Can you work these out from the model? Positions are in its coordinate system, mm. Coordinates: 2 decimals unless noted, no trailing zeros. Write each loop counter-clockwise with the first axis right and the second up, starting at its lowest first coordinate (ties: lowest second). Pieces come first, ordered by that corner, then holes.
```python
from build123d import *

# Parameters (mm, degrees)
SKETCH2_R           = 6.35
SKETCH2_R_2         = 3.175
SKETCH2_R_3         = 10.9855
BOSS_EXTRUDE1_DEPTH = 4.445
SKETCH4_R           = 3.175
CUT_EXTRUDE2_DEPTH  = 148.450257689
SKETCH6_W           = 63.5
SKETCH6_H           = 2.797978373
CUT_EXTRUDE3_DEPTH  = 148.450257689


with BuildPart() as part:
    # Sketch2 → Boss-Extrude1 (new body)
    with BuildSketch(Plane.XY):
        with BuildLine():
            Line((31.75, 112.17275), (-31.75, 112.17275))
            Line((-31.75, 112.17275), (-31.75, 52.48275))
            ThreePointArc((-31.75, 52.48275), (-12.7, -17.145), (-31.75, -86.77275))
            Line((-31.75, -86.77275), (-31.75, -112.17275))
            ThreePointArc((-31.75, -112.17275), (0, -143.92275), (31.75, -112.17275))
            Line((31.75, -112.17275), (31.75, -86.77275))
            ThreePointArc((31.75, -86.77275), (12.7, -17.145), (31.75, 52.48275))
            Line((31.75, 52.48275), (31.75, 112.17275))
        make_face()
        with Locations((0, -112.17275)):
            Circle(SKETCH2_R, mode=Mode.SUBTRACT)
        with Locations((-22.86, 79.15275)):
            Circle(SKETCH2_R_2, mode=Mode.SUBTRACT)
        with Locations((0, 65.18275)):
            Circle(SKETCH2_R_2, mode=Mode.SUBTRACT)
        with Locations((0, 86.77275)):
            Circle(SKETCH2_R_3, mode=Mode.SUBTRACT)
        with Locations((22.86, 79.15275)):
            Circle(SKETCH2_R_2, mode=Mode.SUBTRACT)
    extrude(amount=BOSS_EXTRUDE1_DEPTH)

    # Sketch4 → Cut-Extrude2 (cut, through all)
    with BuildSketch(Plane.XY.offset(4.445)):
        with Locations((0, 42.32275)):
            Circle(SKETCH4_R)
        with Locations((0, -51.21275)):
            Circle(SKETCH4_R)
    extrude(amount=-CUT_EXTRUDE2_DEPTH, mode=Mode.SUBTRACT)

    # Sketch6 → Cut-Extrude3 (cut, through all)
    with BuildSketch(Plane(origin=(0, 0, 0), x_dir=(-1, 0, 0), z_dir=(0, 0, -1))):
        with BuildLine():
            Line((-31.75, 112.17275), (-31.75, 87.727850063))
            Line((-31.75, 87.727850063), (-10.961308866, 102.353257307))
            ThreePointArc((-10.961308866, 102.353257307), (0.491450562, 105.816409741), (11.750340751, 101.767148695))
            Line((11.750340751, 101.767148695), (31.75, 86.094442115))
            Line((31.75, 86.094442115), (31.75, 112.17275))
            Line((31.75, 112.17275), (-31.75, 112.17275))
        make_face()
        with Locations((0, 113.571739187)):
            Rectangle(SKETCH6_W, SKETCH6_H)
    extrude(amount=-CUT_EXTRUDE3_DEPTH, mode=Mode.SUBTRACT)


solid = part.part
```
1. If we section it at C-C, the plane z = 1.4: Count the separate pieces of the cut face and the enclosed holes in it, plus the area to 3 significant figures.
2. If we section it at A-A, the plane x = 0: List the corners of the cut face in (y, z) for me (3 decimals).
3. I'm going to push flat-ended pins straight in: P1, Ø2, axis at x = -24.5, z = 3, coming from the +Y side; P2, Ø7.5, axis at x = 0, y = -112.17, coming from the -Z side. Where does each tip first touch, or does it pass through?
4. We'd pull the mould along Y, two halves only. Please class faces 1 (the face through (-0.32, 105.82, 2.19)), 2 (the face through (31.75, 70, 2)), 3 (the face through (-12.704, -16.122, 2.191)): released by +Y, released by -Y, zero draft, split by the parting line, or undercut.
5. If I drill on L1, parallel to Y at x = 0, z = 0.9; L2, parallel to Y at x = -1, z = 3.05; L3, parallel to Y at x = -24, z = 3.65, over which ranges is the centre line in solid material (lowest first)?
6. If we section it at B-B, the plane x = 23: List the corners of the cut face in (y, z) for me (3 decimals), plus the area to 3 significant figures.
7. If we section it at D-D, the plane x = -17: List the corners of the cut face in (y, z) for me (3 decimals), plus the area to 3 significant figures.
Answers:
1. separate pieces: 1
1. enclosed holes: 7
1. area: 10,700 mm2
2. outline: (-143.923, 0) - (-118.523, 0) - (-118.523, 4.445) - (-143.923, 4.445) - close; (-105.823, 0) - (-54.388, 0) - (-54.388, 4.445) - (-105.823, 4.445) - close; (-48.038, 0) - (39.148, 0) - (39.148, 4.445) - (-48.038, 4.445) - close; (45.498, 0) - (62.008, 0) - (62.008, 4.445) - (45.498, 4.445) - close; (68.358, 0) - (75.787, 0) - (75.787, 4.445) - (68.358, 4.445) - close; (97.758, 0) - (105.823, 0) - (105.823, 4.445) - (97.758, 4.445) - close
3. P1: stops at y = 92.56
3. P2: passes through
4. face 1: released by +Y
4. face 2: zero draft
4. face 3: undercut
5. L1: y = -143.92 to -118.52, -105.82 to -54.39, -48.04 to 39.15, 45.5 to 62.01, 68.36 to 75.79, 97.76 to 105.82
5. L2: y = -143.91 to -118.44, -105.9 to -54.23, -48.2 to 39.31, 45.34 to 62.17, 68.2 to 75.83, 97.71 to 105.8
5. L3: y = -132.96 to -71.58, 37.29 to 76.19, 82.12 to 92.17
6. outline: (-134.06, 0) - (-69.216, 0) - (-69.216, 4.445) - (-134.06, 4.445) - close; (34.926, 0) - (75.981, 0) - (75.981, 4.445) - (34.926, 4.445) - close; (82.325, 0) - (93.884, 0) - (93.884, 4.445) - (82.325, 4.445) - close
6. area: 522 mm2
7. outline: (-138.988, 0) - (-51.17, 0) - (-51.17, 4.445) - (-138.988, 4.445) - close; (16.88, 0) - (97.653, 0) - (97.653, 4.445) - (16.88, 4.445) - close
7. area: 749 mm2
